Autodesk Inventor part; units mm, degrees
ref_plane "YZ Plane" through (0, 0, 0) normal (1, 0, 0) x (0, 1, 0)
ref_plane "XZ Plane" through (0, 0, 0) normal (0, 1, 0) x (-1, 0, 0)
ref_plane "XY Plane" through (0, 0, 0) normal (0, 0, 1) x (1, 0, 0)
sketch "Sketch1" plane through (0, 0, 0) normal (0, 1, 0) x (-1, 0, 0)
  line L0 (40, -60) -> (-40, -60)
  line L1 (-40, -60) -> (-40, 60)
  line L2 (-40, 60) -> (40, 60)
  line L3 (40, 60) -> (40, -60)
  line L4 (5, -5) -> (-5, -5)
  line L5 (-5, -5) -> (-5, 5)
  line L6 (-5, 5) -> (5, 5)
  line L7 (5, 5) -> (5, -5)
  point P0 (0, 0)
  point P1 (-5, 0)
  dimension "d1" = 120
  dimension "d2" = 80
  dimension "d3" = 10
  dimension "d4" = 10
  dimension "d5" = 5
  dimension "d6" = 5
  dimension "d7" = 40
  dimension "d8" = 60
extrude "Extrusion1" add sketch "Sketch1" against normal blind 80
sketch "Sketch5" plane through (40, 0, 60) normal (1, 0, 0) x (0, 0, -1)
  line L0 (120, 0) -> (0, 0)
  line L1 (120, 0) -> (120, -80)
  line L2 (120, -80) -> (0, -80)
  line L3 (0, 0) -> (0, -80)
  point P0 (60, 0)
extrude "Extrusion3" cut sketch "Sketch5" against normal blind 40
properties part number "socket_V2"
Source: CAD feature listing. Evaluate the final solid. Frame: model axes, mm. A direction names the side the tool comes from. Round coordinates to 2 decimals unless told otherwise and drop trailing zeros. Write item = value, one per line. Start each with the question number.
(1) Pin query (flat end, axial travel): pin 1 (5 mm diameter, centred on y = -28.5, z = 1.5, fed in from +X). Return the tip coordinate at first contact, or that it passes through.
(2) Ray query, line 1 along Z through (x, y) = (-2, -71). Return the intervals inside material, ascending. Write a range as from..to.
(3) Pull-direction query (Z, two-part tool) for faces 1 (the face through (-20, -80, 1)), 2 (the face through (-20, -39, -60)), 3 (the face through (-3, -39, -5)); classes: +Z half, -Z half, draft (parallel to the pull), parting line (faces both ways), or undercut.
(4) Set-up query: faces 4 (the face through (-5, -39, 0)), 5 (the face through (-40, -39, 1)). Return all of +Z, -Z, +X, -X, +Y, -Y with unobstructed straight access to the full face (end or side cutting, diameter ignored); none if empty.
Conclusion:
q1.pin_1 = -5
q2.line_1 = -60..-5, 5..60
q3.face_1 = draft
q3.face_2 = -Z half
q3.face_3 = undercut
q4.face_4 = +X, +Y, -Y
q4.face_5 = +Z, -Z, -X, +Y, -Y
